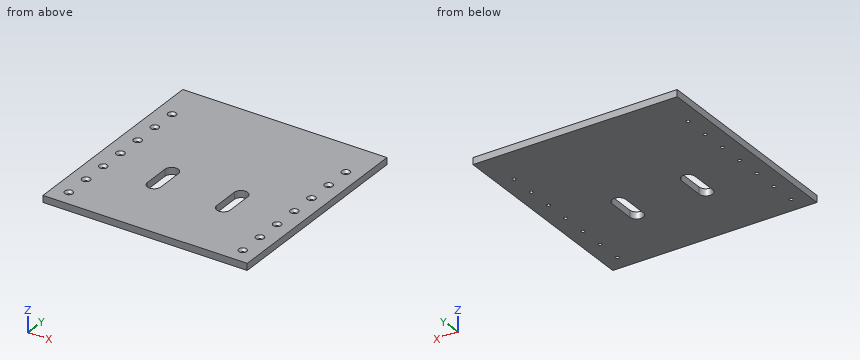
from build123d import *

# Parameters (mm, degrees)
SKETCH1_W                                       = 196.85
SKETCH1_H                                       = 203.2
BOSS_EXTRUDE1_DEPTH                             = 6.604
CUT_EXTRUDE7_DEPTH                              = 313.254468048
SKETCH4_W                                       = 196.85
SKETCH4_H                                       = 0.6096
BOSS_EXTRUDE2_DEPTH                             = 12
SKETCH14_W                                      = 196.85
SKETCH14_H                                      = 11.938
BOSS_EXTRUDE3_DEPTH                             = 6.604
SKETCH13_W                                      = 196.85
SKETCH13_H                                      = 0.6096
CUT_EXTRUDE9_DEPTH                              = 12
CSK_FOR_M3_FLAT_HEAD_MACHINE_SCREW3_D           = 3.4
CSK_FOR_M3_FLAT_HEAD_MACHINE_SCREW3_CSINK_D     = 7.824
CSK_FOR_M3_FLAT_HEAD_MACHINE_SCREW3_CSINK_ANGLE = 90


with BuildPart() as part:
    # Sketch1 → Boss-Extrude1 (new body)
    with BuildSketch(Plane(origin=(0, 0, 0), x_dir=(1, 0, 0), z_dir=(0, 0, -1))):
        with Locations((-104.775, 135.4)):
            Rectangle(SKETCH1_W, SKETCH1_H)
    extrude(amount=BOSS_EXTRUDE1_DEPTH)

    # Sketch2 → Cut-Extrude7 (cut, through all)
    with BuildSketch(Plane(origin=(0, 0, -6.604), x_dir=(1, 0, 0), z_dir=(0, 0, -1))):
        with BuildLine():
            Line((-131.7, 173.5), (-131.7, 148))
            ThreePointArc((-131.7, 148), (-138.2, 141.5), (-144.7, 148))
            Line((-144.7, 148), (-144.7, 173.5))
            ThreePointArc((-144.7, 173.5), (-138.2, 180), (-131.7, 173.5))
        make_face()
        with BuildLine():
            Line((-64.85, 173.5), (-64.85, 148))
            ThreePointArc((-64.85, 148), (-71.35, 141.5), (-77.85, 148))
            Line((-77.85, 148), (-77.85, 173.5))
            ThreePointArc((-77.85, 173.5), (-71.35, 180), (-64.85, 173.5))
        make_face()
    extrude(amount=-CUT_EXTRUDE7_DEPTH, mode=Mode.SUBTRACT)

    # Sketch4 → Boss-Extrude2 (add)
    with BuildSketch(Plane.XY):
        with Locations((-104.706641567, -34.1048)):
            Rectangle(SKETCH4_W, SKETCH4_H)
    extrude(amount=BOSS_EXTRUDE2_DEPTH)

    # Sketch14 → Boss-Extrude3 (add)
    with BuildSketch(Plane.XY):
        with Locations((-104.775, -53.935004147)):
            Rectangle(SKETCH14_W, SKETCH14_H)
    extrude(amount=-BOSS_EXTRUDE3_DEPTH)

    # Sketch13 → Cut-Extrude9 (cut)
    with BuildSketch(Plane.XY.offset(12)):
        with Locations((-104.706641567, -34.1048)):
            Rectangle(SKETCH13_W, SKETCH13_H)
    extrude(amount=-CUT_EXTRUDE9_DEPTH, mode=Mode.SUBTRACT)

    # CSK for M3 Flat Head Machine Screw3 (through all)
    with Locations(Plane.XY):
        with Locations((-188.576641567, -71.467767821), (-188.576641567, -221.467767821), (-188.576641567, -196.467767821), (-188.576641567, -171.467767821), (-188.576641567, -146.467767821), (-188.576641567, -121.467767821), (-188.576641567, -96.467767821)):
            csk_for_m3_flat_head_machine_screw3 = CounterSinkHole(CSK_FOR_M3_FLAT_HEAD_MACHINE_SCREW3_D / 2, CSK_FOR_M3_FLAT_HEAD_MACHINE_SCREW3_CSINK_D / 2, counter_sink_angle=CSK_FOR_M3_FLAT_HEAD_MACHINE_SCREW3_CSINK_ANGLE)

    # Mirror1: CSK for M3 Flat Head Machine Screw3 across plane
    add(csk_for_m3_flat_head_machine_screw3.mirror(Plane.ZY.offset(104.774999995)), mode=Mode.SUBTRACT)


solid = part.part
Model file for the job. Use its own axes, mm. Give positions to 0.01 mm unless a question says otherwise; leave off trailing zeros. Loops run counter-clockwise (first coordinate to the right, second up) from the corner with the lowest first, then second, coordinate; pieces in that order, holes last.
1) Wall check: line 1 (X direction, y = -148.5, z = -3); line 2 (X direction, y = -219.5, z = -1.25); line 3 (Y direction, x = -75, z = -2.25). Give the ranges that are in metal, low to high.
2) Flat gauge pins, fed straight in: pin 1 Ø1.5 at (x, y) = (-135, -130.5) entering from +Z; pin 2 Ø4.5 at (x, y) = (-188.58, -71.47) entering from +Z; pin 3 Ø4 at (x, y) = (-188.58, -196.47) entering from +Z. Where does each tip first touch, or does it go through?
3) Saw through at A-A (x = -138.2). Write the cut outline in (y, z), plus the area to 3 significant figures.
4) Saw through at B-B (z = -5.5). Count the separate pieces of the cut face and the enclosed holes in it, plus the area to 3 significant figures.
Answer block:
1. line 1: x = -203.2 to -144.7, -131.7 to -77.85, -64.85 to -6.35
1. line 2: x = -203.2 to -190.37, -186.78 to -22.77, -19.18 to -6.35
1. line 3: y = -237 to -178.88, -142.62 to -33.8
2. pin 1: stops at z = 0
2. pin 2: stops at z = -1.66
2. pin 3: stops at z = -1.91
3. outline: (-237, -6.6) - (-180, -6.6) - (-180, 0) - (-237, 0) - close; (-141.5, -6.6) - (-33.8, -6.6) - (-33.8, 0) - (-141.5, 0) - close
3. area: 1,090 mm2
4. separate pieces: 1
4. enclosed holes: 16
4. area: 38,900 mm2
